For this review, take the finished solid that the model builds, in its own axes (mm). A direction names the side the tool comes from. Coordinates: 2 decimals unless noted, no trailing zeros. Write each loop counter-clockwise with the first axis right and the second up, starting at its lowest first coordinate (ties: lowest second). Pieces come first, ordered by that corner, then holes. Notation, with made-up numbers: (49.5, 41) -> (66.5, 41) arc R18 ccw to (66.5, 55) -> close; hole circle Ø2 at (70.25, -10). An arc over 180 degrees is marked (long way). One line per item, written item: value. Start each with the question number.
1) Add section A-A (x = 34). State the section outline as (y, z) points, and give its area (3 significant figures).
2) For probe 1 along X at (y, z) = (86.5, 221.5); probe 2 along Z at (x, y) = (128, -24.5); probe 3 along Z at (x, y) = (136, 106), list the stretches that pass through material, from the lowest coordinate up. Write a range as from..to.
3) Add section C-C (z = 183.5). State how many separate pieces and enclosed holes the cut face has, and give its area (3 significant figures).
4) For pin 1 Ø3 at (y, z) = (94.5, 158.5) entering from -X; pin 2 Ø3 at (x, z) = (84, 109) entering from -Y; pin 3 Ø6 at (x, z) = (84, 58) entering from -Y, all flat-tipped, find the tip position at first contact; note any pin that passes through.
5) Mouldability with a two-part tool opening along Y and no side actions: class faces 1 (the flat face through (34.58, 7.62, 171.39)), 2 (the flat face through (84.7, 30.5, 230)), 3 (the flat face through (34.58, 12.19, 169.29)) as released by +Y, released by -Y, zero draft, split by the parting line, or undercut.
6) Add section D-D (x = 171). State the section outline as (y, z) points.
7) Machinability: for faces 4 (the cylindrical face through (197.46, 5.35, 159.88)), 5 (the flat face through (197.46, -8.61, 73.48)), 6 (the flat face through (5, -26, 138)), which of the approach directions +Z, -Z, +X, -X, +Y, -Y give a long, thin tool a straight path to every point of the face, cutting with its end or side? Answer none if there is none.
8) Add section B-B (y = 114). State the section outline as (x, z) points, and give its area (3 significant figures).
from build123d import *

# Parameters (mm, degrees)
P_IDAT_VYSUNUT_M1_DEPTH  = 50
SKICA7_W                 = 200
SKICA7_H                 = 50
P_IDAT_VYSUNUT_M5_DEPTH  = 30
P_IDAT_VYSUNUT_M6_DEPTH  = 5
LINPOLE1_COUNT           = 4
LINPOLE1_PITCH           = 65
P_IDAT_VYSUNUT_M10_DEPTH = 60
LINPOLE3_COUNT           = 3
LINPOLE3_PITCH           = 65
SKICA17_W                = 60
SKICA17_H                = 132.33
ODEBRAT_VYSUNUT_M3_DEPTH = 10
P_IDAT_VYSUNUT_M12_DEPTH = 5
LINPOLE4_COUNT           = 2
LINPOLE4_PITCH           = 65
P_IDAT_VYSUNUT_M13_DEPTH = 60
SKICA20_R                = 2.5
ODEBRAT_VYSUNUT_M4_DEPTH = 10


with BuildPart() as part:
    # Skica1 → Přidat vysunutím1 (new body)
    with BuildSketch(Plane.XY):
        Polygon((0, 0), (200, 0), (200, 350), (70, 220), (0, 220), align=None)
    extrude(amount=P_IDAT_VYSUNUT_M1_DEPTH)

    # Skica7 → Přidat vysunutím5 (add)
    with BuildSketch(Plane.XY.offset(50)):
        with Locations((100, 35)):
            Rectangle(SKICA7_W, SKICA7_H)
    extrude(amount=P_IDAT_VYSUNUT_M5_DEPTH)

    # Skica9 → Přidat vysunutím6 (add)
    with BuildSketch(Plane.ZY):
        with BuildLine():
            Line((80, 10), (66.774778957, -27.75041097))
            Line((66.774778957, -27.75041097), (128.119196783, -49.241395164))
            Line((128.119196783, -49.241395164), (134.731807304, -30.366189679))
            ThreePointArc((134.731807304, -30.366189679), (160.364777666, 5.738922578), (201.274673199, 22.680255114))
            Line((201.274673199, 22.680255114), (230, 25.917114128))
            Line((230, 25.917114128), (230, 105.917114128))
            Line((230, 105.917114128), (100, 60))
            Line((100, 60), (80, 60))
            Line((80, 60), (80, 10))
        make_face()
    p_idat_vysunut_m6 = extrude(amount=-P_IDAT_VYSUNUT_M6_DEPTH)

    # LinPole1: Přidat vysunutím6 ×4
    with Locations(*[(i * LINPOLE1_PITCH, 0, 0) for i in range(1, LINPOLE1_COUNT)]):
        add(p_idat_vysunut_m6)

    # Skica12 → Přidat vysunutím10 (add)
    with BuildSketch(Plane(origin=(5, 0, 0), x_dir=(0, 0, -1), z_dir=(1, 0, 0))):
        Polygon((-230, 105.917114128), (-230, 100.61438772), (-105.220267206, 56.541116708), (-71.496803297, -29.404692713), (-66.774778957, -27.75041097), (-101.40042077, 60.494640618), align=None)
        Polygon((-230, 25.917114128), (-230, 30.952852669), (-193.421577993, 26.571602615), (-144.481791005, -2.596155027), (-123.37587339, -47.579651656), (-128.119196783, -49.241395164), (-148.357587613, -6.10687705), (-195.069843452, 21.733288203), align=None)
    p_idat_vysunut_m10 = extrude(amount=P_IDAT_VYSUNUT_M10_DEPTH)

    # LinPole3: Přidat vysunutím10 ×3
    with Locations(*[(i * LINPOLE3_PITCH, 0, 0) for i in range(1, LINPOLE3_COUNT)]):
        add(p_idat_vysunut_m10)

    # Skica17 → Odebrat vysunutím3 (cut)
    with BuildSketch(Plane(origin=(0, 21.941769172, -7.750020917), x_dir=(1, 0, 0), z_dir=(0, 0.9429111773554218, -0.33304430879120595))):
        with Locations((165, -185.979662856)):
            Rectangle(SKICA17_W, SKICA17_H)
    extrude(amount=-ODEBRAT_VYSUNUT_M3_DEPTH, mode=Mode.SUBTRACT)

    # Skica18 → Přidat vysunutím12 (add)
    with BuildSketch(Plane(origin=(135, 0, 0), x_dir=(0, 0, -1), z_dir=(1, 0, 0))):
        Polygon((-101.40042077, 60.494640618), (-227.071424446, 195.869453982), (-230, 105.917114128), align=None)
    p_idat_vysunut_m12 = extrude(amount=-P_IDAT_VYSUNUT_M12_DEPTH)

    # LinPole4: Přidat vysunutím12 ×2
    with Locations(*[(i * LINPOLE4_PITCH, 0, 0) for i in range(1, LINPOLE4_COUNT)]):
        add(p_idat_vysunut_m12)

    # Skica19 → Přidat vysunutím13 (add)
    with BuildSketch(Plane(origin=(135, 0, 0), x_dir=(0, 0, -1), z_dir=(1, 0, 0))):
        Polygon((-227.071424446, 195.869453982), (-101.40042077, 60.494640618), (-105.224563901, 61.845360745), (-227.158510983, 193.194557029), align=None)
    extrude(amount=P_IDAT_VYSUNUT_M13_DEPTH)

    # Skica20 → Odebrat vysunutím4 (cut)
    with BuildSketch(Plane.XY.offset(50)):
        with Locations((50.459484354, 160.603206666)):
            Circle(SKICA20_R)
    extrude(amount=-ODEBRAT_VYSUNUT_M4_DEPTH, mode=Mode.SUBTRACT)


solid = part.part
Numbers:
1. outline: (-49.24, 128.12) -> (-47.58, 123.38) -> (-2.6, 144.48) -> (26.57, 193.42) -> (30.95, 230) -> (25.92, 230) -> (21.73, 195.07) -> (-6.11, 148.36) -> close; (-29.4, 71.5) -> (-27.75, 66.77) -> (60.49, 101.4) -> (105.92, 230) -> (100.61, 230) -> (56.54, 105.22) -> close; (0, 0) -> (220, 0) -> (220, 50) -> (60, 50) -> (60, 80) -> (10, 80) -> (10, 50) -> (0, 50) -> close
1. area: 14,300 mm²
2. probe 1: 0..5, 65..70, 130..135, 195..200
2. probe 2: 68.05..73.42, 134.2..139.73
2. probe 3: 0..50, 143.64..146.21
3. separate pieces: 1
3. enclosed holes: 3
3. area: 3,860 mm²
4. pin 1: x = 130
4. pin 2: y = 57.35
4. pin 3: y = 10
5. face 1: released by -Y
5. face 2: zero draft
5. face 3: undercut
6. outline: (-49.24, 128.12) -> (-47.58, 123.38) -> (-2.6, 144.48) -> (26.57, 193.42) -> (30.95, 230) -> (25.92, 230) -> (21.73, 195.07) -> (-6.11, 148.36) -> close; (-29.4, 71.5) -> (-27.75, 66.77) -> (60.49, 101.4) -> (195.87, 227.07) -> (193.19, 227.16) -> (61.85, 105.22) -> (57.13, 106.89) -> (56.54, 105.22) -> close; (0, 0) -> (321, 0) -> (321, 50) -> (60, 50) -> (60, 80) -> (10, 80) -> (10, 50) -> (0, 50) -> close
7. face 4: +Z, +X, -Y
7. face 5: +X, -X
7. face 6: +Z, -X, -Y
8. outline: (0, 0) -> (200, 0) -> (200, 50) -> (0, 50) -> close; (130, 151.07) -> (200, 151.07) -> (200, 229.74) -> (195, 229.74) -> (195, 153.64) -> (135, 153.64) -> (135, 229.74) -> (130, 229.74) -> close
8. area: 10,900 mm²
